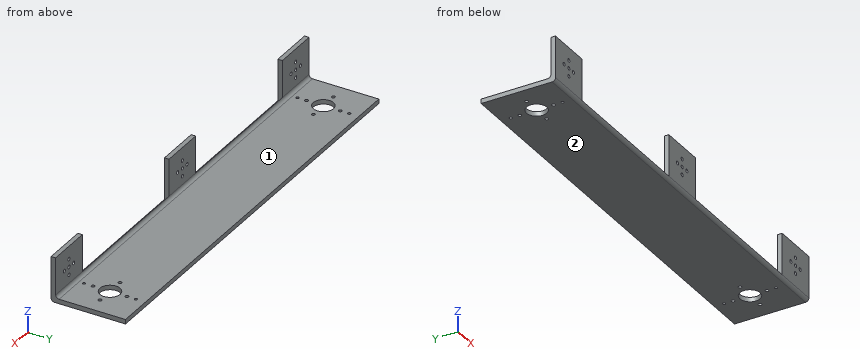
from build123d import *

# Parameters (mm, degrees)
BOSS_EXTRUDE1_DEPTH = 380
FILLET4_R           = 3
HOLE2_D             = 18
HOLE2_DEPTH         = 4
SKETCH18_W          = 130
SKETCH18_H          = 37
CUT_EXTRUDE1_DEPTH  = 4
HOLE5_D             = 3
HOLE5_DEPTH         = 4
HOLE6_D             = 3
HOLE6_DEPTH         = 4
HOLE7_D             = 2.5
HOLE7_DEPTH         = 4
SKETCH27_R          = 1.55
CUT_EXTRUDE3_DEPTH  = 4


with BuildPart() as part:
    # Sketch1 → Boss-Extrude1 (new body)
    with BuildSketch(Plane(origin=(0, 0, 0), x_dir=(0, 0, -1), z_dir=(1, 0, 0))):
        Polygon((-32.21677116, -27.719218501), (7.78322884, -27.719218501), (7.78322884, 38.280781499), (3.78322884, 38.280781499), (3.78322884, -23.719218501), (-32.21677116, -23.719218501), align=None)
    extrude(amount=BOSS_EXTRUDE1_DEPTH)

    # Fillet4
    fillet4_edges = [part.edges().sort_by_distance(p)[0] for p in [
        (190, -23.719218501, -3.78322884),
        (190, -27.719218501, -7.78322884),
    ]]
    fillet(fillet4_edges, radius=FILLET4_R)

    # Hole2
    with Locations(Plane.XY.offset(-3.78322884)):
        with Locations((30, 6.780781499), (350, 6.780781499)):
            Hole(HOLE2_D / 2, depth=HOLE2_DEPTH)

    # Sketch18 → Cut-Extrude1 (cut)
    with BuildSketch(Plane.XZ.offset(27.719218501)):
        with Locations((105, 13.71677116)):
            Rectangle(SKETCH18_W, SKETCH18_H)
        with Locations((275, 13.71677116)):
            Rectangle(SKETCH18_W, SKETCH18_H)
    extrude(amount=-CUT_EXTRUDE1_DEPTH, mode=Mode.SUBTRACT)

    # Hole5
    with Locations(Plane(origin=(360, -27.719218501, 13.71677116), x_dir=(0, 0, -1), z_dir=(0, -1, 0))):
        with Locations((0, 0), (0, -170), (0, -340)):
            Hole(HOLE5_D / 2, depth=HOLE5_DEPTH)

    # Hole6
    with Locations(Plane(origin=(30, 21.780781499, -7.78322884), x_dir=(-1, 0, 0), z_dir=(0, 0, -1))):
        with Locations((0, 0), (15, -15), (0, -30), (-320, -30), (-335, -15), (-320, 0), (-305, -15), (-15, -15)):
            Hole(HOLE6_D / 2, depth=HOLE6_DEPTH)

    # Hole7
    with Locations(Plane(origin=(30, 29.780781499, -7.78322884), x_dir=(-1, 0, 0), z_dir=(0, 0, -1))):
        with Locations((0, 0), (0, -46), (-320, 0), (-320, -46)):
            Hole(HOLE7_D / 2, depth=HOLE7_DEPTH)

    # Sketch27 → Cut-Extrude3 (cut)
    with BuildSketch(Plane(origin=(0, -23.719218501, 0), x_dir=(1, 0, 0), z_dir=(0, 1, 0))):
        with Locations((20, -20.71677116)):
            Circle(SKETCH27_R)
        with Locations((13, -13.71677116)):
            Circle(SKETCH27_R)
        with Locations((20, -6.71677116)):
            Circle(SKETCH27_R)
        with Locations((27, -13.71677116)):
            Circle(SKETCH27_R)
        with Locations((360, -20.71677116)):
            Circle(SKETCH27_R)
        with Locations((353, -13.71677116)):
            Circle(SKETCH27_R)
        with Locations((360, -6.71677116)):
            Circle(SKETCH27_R)
        with Locations((367, -13.71677116)):
            Circle(SKETCH27_R)
        with Locations((190, -20.71677116)):
            Circle(SKETCH27_R)
        with Locations((183, -13.71677116)):
            Circle(SKETCH27_R)
        with Locations((190, -6.71677116)):
            Circle(SKETCH27_R)
        with Locations((197, -13.71677116)):
            Circle(SKETCH27_R)
    extrude(amount=-CUT_EXTRUDE3_DEPTH, mode=Mode.SUBTRACT)


solid = part.part
Read the model definition and answer for the solid it produces. Units are mm, in the model's axes. Face numbers are marked on the shaded views. A direction names the side the tool comes from. Give positions to 0.01 mm unless a question says otherwise; leave off trailing zeros. Write each loop counter-clockwise with the first axis right and the second up, starting at its lowest first coordinate (ties: lowest second). Pieces come first, ordered by that corner, then holes. Notation, with made-up numbers: (45.5, 65.25) - (54.5, 65.25) arc R13 cw to (54.5, 81.25) - close; hole circle Ø8 at (88.25, 51.5). An arc over 180 degrees is marked (long way). Answer in a Markdown table with one row per item. Add a question column.
Item 1: Flat-ended cylindrical pins translate along their axes: P1, Ø2.5, axis at x = 350, y = -8.22, coming from the +Z side; P2, Ø5, axis at x = 45, y = 6.78, coming from the -Z side; P3, Ø10, axis at x = 356.5, z = 13, coming from the +Y side; P4, Ø10, axis at x = 186.5, y = -13.5, coming from the +Z side. Find the tip coordinate at first contact, or state that the pin passes through.
Item 2: Section A-A, the plane x = 35.5 is taken. Write down the section's boundary in (y, z), and give its area (3 significant figures).
Item 3: Find the intervals of material crossed by L1, parallel to X at y = 30, z = -5; L2, parallel to X at y = 21, z = -4.5; L3, parallel to Y at x = 30, z = -6.9, in increasing order.
Item 4: Section B-B, the plane x = 313 is taken. Write down the section's boundary in (y, z), and give its area (3 significant figures).
Item 5: A tool of negligible diameter and unlimited length cuts with its end or side. For the marked faces 1 and 2, from which of +Z, -Z, +X, -X, +Y, -Y can it reach the whole face along a straight path? Write none if from no direction.
Recorded:
| question | item | result |
|---|---|---|
| 1 | P1 | passes through |
| 1 | P2 | stops at z = -7.78 |
| 1 | P3 | stops at y = -23.72 |
| 1 | P4 | stops at z = -3.78 |
| 2 | outline | (-27.72, -4.78) arc R3 ccw to (-24.72, -7.78) - (-0.34, -7.78) - (-0.34, -3.78) - (-20.72, -3.78) arc R3 cw to (-23.72, -0.78) - (-23.72, 32.22) - (-27.72, 32.22) - close; (13.9, -7.78) - (38.28, -7.78) - (38.28, -3.78) - (13.9, -3.78) - close |
| 2 | area | 351 mm2 |
| 3 | L1 | x = 0 to 28.77, 31.23 to 348.77, 351.23 to 380 |
| 3 | L2 | x = 0 to 28.72, 31.28 to 348.72, 351.28 to 380 |
| 3 | L3 | y = -26.85 to -17.47, -14.97 to -9.72, -6.72 to -2.22, 15.78 to 20.28, 23.28 to 28.53, 31.03 to 38.28 |
| 4 | outline | (-27.72, -4.78) arc R3 ccw to (-24.72, -7.78) - (38.28, -7.78) - (38.28, -3.78) - (-20.72, -3.78) arc R3 cw to (-23.72, -0.78) - (-23.72, -4.78) - close |
| 4 | area | 260 mm2 |
| 5 | face 1 | +Z, +X, -X, +Y |
| 5 | face 2 | -Z, +X, -X, +Y, -Y |
